from build123d import *

# Parameters (mm, degrees)
SKETCH1_W           = 254
SKETCH1_H           = 127
BOSS_EXTRUDE2_DEPTH = 19.05
SKETCH2_W           = 244
SKETCH2_H           = 117
CUT_EXTRUDE1_DEPTH  = 17.05
SKETCH4_W           = 70
SKETCH4_H           = 127
CUT_EXTRUDE2_DEPTH  = 44
SKETCH6_W           = 5
SKETCH6_H           = 117
BOSS_EXTRUDE3_DEPTH = 17.05
SKETCH9_W           = 174
SKETCH9_H           = 117
BOSS_EXTRUDE4_DEPTH = 4
SKETCH12_W          = 8.5
SKETCH12_H          = 5
CUT_EXTRUDE3_DEPTH  = 13.05
CUT_EXTRUDE4_DEPTH  = 1
CUT_EXTRUDE5_DEPTH  = 4.5
SKETCH17_W          = 2.2
SKETCH17_H          = 51.1
CUT_EXTRUDE6_DEPTH  = 1.5
SKETCH19_W          = 7.4
SKETCH19_H          = 6
CUT_EXTRUDE7_DEPTH  = 4
SKETCH20_R          = 3.5
CUT_EXTRUDE8_DEPTH  = 2.5
SKETCH23_R          = 1.5
CUT_EXTRUDE9_DEPTH  = 38
BOSS_EXTRUDE5_DEPTH = 13.05
SKETCH25_W          = 9.3
SKETCH25_H          = 6
CUT_EXTRUDE10_DEPTH = 4
SKETCH26_W          = 8.5
SKETCH26_H          = 1.89071474
CUT_EXTRUDE11_DEPTH = 3.5
SKETCH27_R          = 0.95
CUT_EXTRUDE13_DEPTH = 25
SKETCH28_R          = 2.06
CUT_EXTRUDE18_DEPTH = 1.24
BOSS_EXTRUDE6_START = 2
SKETCH31_W          = 184
SKETCH31_H          = 127
SKETCH31_R          = 2.06
SKETCH31_R_2        = 3.5
BOSS_EXTRUDE6_DEPTH = 2
CUT_EXTRUDE19_REACH = 145.542
SKETCH14_W          = 11.462803728
SKETCH14_H          = 5


with BuildPart() as part:
    # Sketch1 → Boss-Extrude2 (new body)
    with BuildSketch(Plane(origin=(0, 0, 0), x_dir=(1, 0, 0), z_dir=(0, 1, 0))):
        Rectangle(SKETCH1_W, SKETCH1_H)
    extrude(amount=BOSS_EXTRUDE2_DEPTH)

    # Sketch2 → Cut-Extrude1 (cut)
    with BuildSketch(Plane.XZ):
        Rectangle(SKETCH2_W, SKETCH2_H)
    extrude(amount=-CUT_EXTRUDE1_DEPTH, mode=Mode.SUBTRACT)

    # Sketch4 → Cut-Extrude2 (cut)
    with BuildSketch(Plane(origin=(0, 19.05, 0), x_dir=(1, 0, 0), z_dir=(0, 1, 0))):
        with Locations((-92, 0)):
            Rectangle(SKETCH4_W, SKETCH4_H)
    extrude(amount=-CUT_EXTRUDE2_DEPTH, mode=Mode.SUBTRACT)

    # Sketch6 → Boss-Extrude3 (add)
    with BuildSketch(Plane.XZ.offset(-17.05)):
        with Locations((-54.5, 0)):
            Rectangle(SKETCH6_W, SKETCH6_H)
    extrude(amount=BOSS_EXTRUDE3_DEPTH)

    # Sketch9 → Boss-Extrude4 (add)
    with BuildSketch(Plane.XZ.offset(-17.05)):
        with Locations((35, 0)):
            Rectangle(SKETCH9_W, SKETCH9_H)
    extrude(amount=BOSS_EXTRUDE4_DEPTH)

    # Sketch12 → Cut-Extrude3 (cut)
    with BuildSketch(Plane.XZ):
        with Locations((35, 61)):
            Rectangle(SKETCH12_W, SKETCH12_H)
    extrude(amount=-CUT_EXTRUDE3_DEPTH, mode=Mode.SUBTRACT)

    # Sketch13 → Cut-Extrude4 (cut)
    with BuildSketch(Plane.XZ.offset(-13.05)):
        Polygon((30.75, 58.5), (24.45, 58.5), (24.45, 7.4), (45.55, 7.4), (45.55, 58.5), (39.25, 58.5), (39.25, 54), (30.75, 54), align=None)
    extrude(amount=-CUT_EXTRUDE4_DEPTH, mode=Mode.SUBTRACT)

    # Sketch15 → Cut-Extrude5 (cut)
    with BuildSketch(Plane.XZ.offset(-13.05)):
        Polygon((30.75, 54), (39.25, 54), (39.25, 58.5), (39.25, 63.5), (30.75, 63.5), (30.75, 58.5), align=None)
    extrude(amount=-CUT_EXTRUDE5_DEPTH, mode=Mode.SUBTRACT)

    # Sketch17 → Cut-Extrude6 (cut)
    with BuildSketch(Plane.XZ.offset(-14.05)):
        with Locations((25.55, 32.95)):
            Rectangle(SKETCH17_W, SKETCH17_H)
        with Locations((44.45, 32.95)):
            Rectangle(SKETCH17_W, SKETCH17_H)
    extrude(amount=-CUT_EXTRUDE6_DEPTH, mode=Mode.SUBTRACT)

    # Sketch19 → Cut-Extrude7 (cut)
    with BuildSketch(Plane.XZ.offset(-14.05)):
        with Locations((30.35, 46.5)):
            Rectangle(SKETCH19_W, SKETCH19_H)
    extrude(amount=-CUT_EXTRUDE7_DEPTH, mode=Mode.SUBTRACT)

    # Sketch20 → Cut-Extrude8 (cut)
    with BuildSketch(Plane(origin=(0, 19.05, 0), x_dir=(1, 0, 0), z_dir=(0, 1, 0))):
        with Locations(Location((-52, -58.5, 0), (0, 0, 270))):
            Circle(SKETCH20_R)
        with Locations(Location((122, -58.5, 0), (0, 0, 270))):
            Circle(SKETCH20_R)
        with Locations(Location((122, 58.5, 0), (0, 0, 270))):
            Circle(SKETCH20_R)
        with Locations(Location((-52, 58.5, 0), (0, 0, 270))):
            Circle(SKETCH20_R)
    extrude(amount=-CUT_EXTRUDE8_DEPTH, mode=Mode.SUBTRACT)

    # Sketch23 → Cut-Extrude9 (cut)
    with BuildSketch(Plane(origin=(0, 16.55, 0), x_dir=(1, 0, 0), z_dir=(0, 1, 0))):
        with Locations(Location((-52, 58.5, 0), (0, 0, 270))):
            Circle(SKETCH23_R)
        with Locations(Location((-52, -58.5, 0), (0, 0, 270))):
            Circle(SKETCH23_R)
        with Locations(Location((122, -58.5, 0), (0, 0, 270))):
            Circle(SKETCH23_R)
        with Locations(Location((122, 58.5, 0), (0, 0, 270))):
            Circle(SKETCH23_R)
    extrude(amount=-CUT_EXTRUDE9_DEPTH, mode=Mode.SUBTRACT)

    # Sketch24 → Boss-Extrude5 (add)
    with BuildSketch(Plane.XZ.offset(-13.05)):
        with BuildLine():
            Line((-52, 57), (-52, 55))
            ThreePointArc((-52, 55), (-49.525126266, 56.025126266), (-48.5, 58.5))
            Line((-48.5, 58.5), (-50.5, 58.5))
            ThreePointArc((-50.5, 58.5), (-50.939339828, 57.439339828), (-52, 57))
        make_face()
        with BuildLine():
            Line((-48.5, -58.5), (-50.5, -58.5))
            ThreePointArc((-50.5, -58.5), (-50.939339828, -57.439339828), (-52, -57))
            Line((-52, -57), (-52, -55))
            ThreePointArc((-52, -55), (-49.525126266, -56.025126266), (-48.5, -58.5))
        make_face()
        with BuildLine():
            Line((122, 55), (122, 57))
            ThreePointArc((122, 57), (120.939339828, 57.439339828), (120.5, 58.5))
            Line((120.5, 58.5), (118.5, 58.5))
            ThreePointArc((118.5, 58.5), (119.525126266, 56.025126266), (122, 55))
        make_face()
        with BuildLine():
            Line((122, -57), (122, -55))
            ThreePointArc((122, -55), (119.525126266, -56.025126266), (118.5, -58.5))
            Line((118.5, -58.5), (120.5, -58.5))
            ThreePointArc((120.5, -58.5), (120.939339828, -57.439339828), (122, -57))
        make_face()
    extrude(amount=BOSS_EXTRUDE5_DEPTH)

    # Sketch25 → Cut-Extrude10 (cut)
    with BuildSketch(Plane.XZ.offset(-14.05)):
        with Locations((38.7, 46.5)):
            Rectangle(SKETCH25_W, SKETCH25_H)
    extrude(amount=-CUT_EXTRUDE10_DEPTH, mode=Mode.SUBTRACT)

    # Sketch26 → Cut-Extrude11 (cut)
    with BuildSketch(Plane.XZ.offset(-14.05)):
        with Locations((35, 53.05464263)):
            Rectangle(SKETCH26_W, SKETCH26_H)
    extrude(amount=-CUT_EXTRUDE11_DEPTH, mode=Mode.SUBTRACT)

    # Sketch27 → Cut-Extrude13 (cut)
    with BuildSketch(Plane.XZ.offset(-14.05)):
        with Locations(Location((40.7, 9.4, 0), (0, 0, 270))):
            Circle(SKETCH27_R)
        with Locations(Location((29.3, 56.5, 0), (0, 0, 270))):
            Circle(SKETCH27_R)
    extrude(amount=-CUT_EXTRUDE13_DEPTH, mode=Mode.SUBTRACT)

    # Sketch28 → Cut-Extrude18 (cut)
    with BuildSketch(Plane(origin=(0, 19.05, 0), x_dir=(1, 0, 0), z_dir=(0, 1, 0))):
        with Locations(Location((40.7, -9.4, 0), (0, 0, 270))):
            Circle(SKETCH28_R)
        with Locations(Location((29.3, -56.5, 0), (0, 0, 270))):
            Circle(SKETCH28_R)
    extrude(amount=-CUT_EXTRUDE18_DEPTH, mode=Mode.SUBTRACT)

    # Sketch31 → Boss-Extrude6 (add)
    with BuildSketch(Plane(origin=(0, 19.05, 0), x_dir=(1, 0, 0), z_dir=(0, 1, 0)).offset(BOSS_EXTRUDE6_START)):
        with Locations((35, 0)):
            Rectangle(SKETCH31_W, SKETCH31_H)
        with Locations(Location((40.7, -9.4, 0), (0, 0, 270))):
            Circle(SKETCH31_R, mode=Mode.SUBTRACT)
        with Locations(Location((-52, 58.5, 0), (0, 0, 270))):
            Circle(SKETCH31_R_2, mode=Mode.SUBTRACT)
        with Locations(Location((-52, -58.5, 0), (0, 0, 270))):
            Circle(SKETCH31_R_2, mode=Mode.SUBTRACT)
        with Locations(Location((29.3, -56.5, 0), (0, 0, 270))):
            Circle(SKETCH31_R, mode=Mode.SUBTRACT)
        with Locations(Location((122, -58.5, 0), (0, 0, 270))):
            Circle(SKETCH31_R_2, mode=Mode.SUBTRACT)
        with Locations(Location((122, 58.5, 0), (0, 0, 270))):
            Circle(SKETCH31_R_2, mode=Mode.SUBTRACT)
    extrude(amount=-BOSS_EXTRUDE6_DEPTH)

    # Cut-Extrude19: up to this face of the body (flat: up to its plane)
    cut_extrude19_end = Plane(part.part.faces().sort_by_distance((35, 17.55, 57.80464263))[0])
    # Sketch14 → Cut-Extrude19 (cut, up to the picked face)
    with BuildSketch(Plane.XZ, mode=Mode.PRIVATE) as cut_extrude19_sk1:
        with Locations((35, 61)):
            Rectangle(SKETCH14_W, SKETCH14_H)
    cut_extrude19_tool1 = split(extrude(cut_extrude19_sk1.sketch, amount=-CUT_EXTRUDE19_REACH, mode=Mode.PRIVATE), bisect_by=cut_extrude19_end, keep=Keep.BOTH, mode=Mode.PRIVATE)
    add(cut_extrude19_tool1.solids().sort_by(Axis((35, 0, 61), (0, 1, 0)))[0], mode=Mode.SUBTRACT)


solid = part.part
Read the model definition and answer for the solid it produces. Units are mm, in the model's axes. A direction names the side the tool comes from. Round coordinates to 2 decimals unless told otherwise and drop trailing zeros. Loops run counter-clockwise (first coordinate to the right, second up) from the corner with the lowest first, then second, coordinate; pieces in that order, holes last. Notation, with made-up numbers: (88.5, -3.75) - (107.5, -3.75) arc R23 cw to (107.5, 25.25) - close; hole circle Ø1 at (-3, 57). An arc over 180 degrees is marked (long way). One line per question, with ' | ' between items. Start each with the question number.
Q1. Section C-C on x = -13 is taken. Give the vertices of the cut face in (y, z).
Q2. Flat-ended cylindrical pins translate along their axes: pin 1 (1 mm diameter, centred on x = 48, z = -9, fed in from -Y); pin 2 (2.5 mm diameter, centred on x = 40.7, z = 9.4, fed in from +Y); pin 3 (2 mm diameter, centred on x = 38.5, y = 15, fed in from +Z). Find the tip coordinate at first contact, or state that the pin passes through.
Q3. Section A-A on y = 8.5 is taken. Give the vertices of the cut face in (x, z), plus the area to 3 significant figures.
Q4. Section D-D on x = 34 is taken. Give the vertices of the cut face in (y, z).
Q5. For faces 1 (the flat face through (28, 0, 61)), 2 (the flat face through (35, 14.05, 26)), 3 (the cylindrical face through (119.9, 18.8, 55.7)), determine the directions among +Z, -Z, +X, -X, +Y, -Y from which every point of the face is accessible in a straight line to the end or side of a thin tool.
Q6. Section B-B on z = -46.5 is taken. Give the vertices of the cut face in (x, y), plus the area to 3 significant figures.
Q7. For a pull along Z with two mould halves and no side action, classify faces 4 (the flat face through (34, 18, 63.5)), 5 (the flat face through (39.25, 16, 55)), 6 (the flat face through (-10, 6, 58.5)) as +Z half, -Z half, draft (parallel to the pull), parting line (faces both ways), or undercut.
Q8. Find the intervals of material crossed by L1, parallel to X at y = 8.5, z = 52.5; L2, parallel to Z at x = 6.5, y = 9.75; L3, parallel to Y at x = 104.5, z = 0.5, in increasing order.
Established:
1) outline: (0, -63.5) - (21.05, -63.5) - (21.05, 63.5) - (0, 63.5) - (0, 58.5) - (13.05, 58.5) - (13.05, -58.5) - (0, -58.5) - close
2) pin 1: y = 13.05 | pin 2: y = 17.81 | pin 3: z = 58.5
3) outline: (-57, -63.5) - (127, -63.5) - (127, 63.5) - (40.73, 63.5) - (40.73, 58.5) - (118.5, 58.5) arc R3.5 ccw to (122, 55) - (122, -55) arc R3.5 ccw to (118.5, -58.5) - (-48.5, -58.5) arc R3.5 ccw to (-52, -55) - (-52, 55) arc R3.5 ccw to (-48.5, 58.5) - (29.27, 58.5) - (29.27, 63.5) - (-57, 63.5) - close; hole circle Ø3 at (-52, -58.5); hole circle Ø3 at (-52, 58.5); hole circle Ø3 at (122, -58.5); hole circle Ø3 at (122, 58.5) | area: 2,960 mm²
4) outline: (0, -63.5) - (21.05, -63.5) - (21.05, 63.5) - (17.55, 63.5) - (17.55, 52.11) - (14.05, 52.11) - (14.05, 49.5) - (18.05, 49.5) - (18.05, 43.5) - (14.05, 43.5) - (14.05, 7.4) - (13.05, 7.4) - (13.05, -58.5) - (0, -58.5) - close
5) face 1: +Z, -Z, +X, -X, -Y | face 2: -Y | face 3: +Y
6) outline: (-57, 0) - (-52, 0) - (-52, 13.05) - (122, 13.05) - (122, 0) - (127, 0) - (127, 21.05) - (-57, 21.05) - close | area: 1,600 mm²
7) face 4: +Z half | face 5: draft | face 6: undercut
8) L1: -57 to -52, 122 to 127 | L2: -63.5 to -58.5, 58.5 to 63.5 | L3: 13.05 to 21.05
